Here's how the part is built. I have some questions about the finished solid (model axes, mm). A direction names the side the tool comes from. Round coordinates to 2 decimals unless told otherwise and drop trailing zeros. Write each loop counter-clockwise with the first axis right and the second up, starting at its lowest first coordinate (ties: lowest second). Pieces come first, ordered by that corner, then holes. Notation, with made-up numbers: M 53.25,-37.5 L 59.25,-37.5 A30 cw 59.25,-12.5 Z; hole C 20.5,-3.75 d8. An arc over 180 degrees is marked long. Use one line per item in the form item = value. Start each with the question number.
Q1. I want a section at A-A on z = -9.5. State how many separate pieces and enclosed holes the cut face has, and give its area (3 significant figures).
Q2. We'd pull the mould along Y, two halves only. Please class faces 3 (the face through (-16, 20, -6.35)), 4 (the face through (49.88, 16.57, -4.47)), 5 (the face through (-107.95, -1, 0)), 6 (the face through (-2, 38.1, 0)): +Y half, -Y half, draft (parallel to the pull), parting line (faces both ways), or undercut.
Q3. I want a section at C-C on x = 21. List the corners of the cut face in (y, z) for me (3 decimals), and give its area (3 significant figures).
Q4. I'm going to push flat-ended pins straight in: pin 1 Ø8.5 at (x, y) = (-56.11, -22.45) entering from +Z; pin 2 Ø15.5 at (x, y) = (47, 12.5) entering from -Z. Where does each tip first touch, or does it pass through?
Q5. I want a section at B-B on x = 95.25. List the corners of the cut face in (y, z) for me, and give its area (3 significant figures).
Q6. I want a section at D-D on y = -25.4. List the corners of the cut face in (x, z) for me, and give its area (3 significant figures).
Q7. For faces 1 (the face through (4.58, -29.31, -9.48)), 2 (the face through (89.384, 22.968, -0.178)), which set-ups out of +Z, -Z, +X, -X, +Y, -Y let a thin tool reach every point of the face, with its end or its side?
Q8. I need wall thicknesses on line 1 along X through (y, z) = (-8, -5.25); line 2 along X through (y, z) = (8, -2.5); line 3 along X through (y, z) = (-25.5, -2.5). Which ranges of each line are inside material? Lowest first, please. Write a range as from..to.
```python
from build123d import *

# Parameters (mm, degrees)
SKETCH1_W           = 215.9
SKETCH1_H           = 76.2
BOSS_EXTRUDE1_DEPTH = 12.7
SKETCH2_R           = 5.159375
SKETCH2_R_2         = 6.985
BOSS_EXTRUDE2_DEPTH = 9.525
SKETCH3_R           = 5.159375
BOSS_EXTRUDE3_DEPTH = 9.525
CUT_EXTRUDE1_DEPTH  = 3.81
LPATTERN1_COUNT     = 2
LPATTERN1_PITCH     = 67.31
SKETCH5_R           = 13.335
CUT_EXTRUDE2_DEPTH  = 2.54
SKETCH6_R           = 6.35
CUT_EXTRUDE3_DEPTH  = 118.260276735
SKETCH7_R           = 20.6502
CUT_EXTRUDE4_DEPTH  = 116.571744492


with BuildPart() as part:
    # Sketch1 → Boss-Extrude1 (new, symmetric)
    with BuildSketch(Plane.XY):
        Rectangle(SKETCH1_W, SKETCH1_H)
        with BuildLine():
            ThreePointArc((-52.148499203, -31.128702045), (-62.84981265, -29.19481265), (-64.783702045, -18.493499203))
            Line((-64.783702045, -18.493499203), (-52.443985877, 8.56765836))
            ThreePointArc((-52.443985877, 8.56765836), (-48.256896453, 14.601896453), (-42.22265836, 18.788985877))
            Line((-42.22265836, 18.788985877), (-15.161500797, 31.128702045))
            ThreePointArc((-15.161500797, 31.128702045), (-6.045595474, 30.472789203), (-1.666659697, 22.450640303))
            ThreePointArc((-1.666659697, 22.450640303), (-1.884046645, 20.42592158), (-2.526297955, 18.493499203))
            Line((-2.526297955, 18.493499203), (-14.866014123, -8.56765836))
            ThreePointArc((-14.866014123, -8.56765836), (-19.053103547, -14.601896453), (-25.08734164, -18.788985877))
            Line((-25.08734164, -18.788985877), (-52.148499203, -31.128702045))
        make_face(mode=Mode.SUBTRACT)
        with BuildLine():
            Line((64.783702045, 18.493499203), (52.443985877, -8.56765836))
            ThreePointArc((52.443985877, -8.56765836), (48.256896453, -14.601896453), (42.22265836, -18.788985877))
            Line((42.22265836, -18.788985877), (15.161500797, -31.128702045))
            ThreePointArc((15.161500797, -31.128702045), (4.46018735, -29.19481265), (2.526297955, -18.493499203))
            Line((2.526297955, -18.493499203), (14.866014123, 8.56765836))
            ThreePointArc((14.866014123, 8.56765836), (19.053103547, 14.601896453), (25.08734164, 18.788985877))
            Line((25.08734164, 18.788985877), (52.148499203, 31.128702045))
            ThreePointArc((52.148499203, 31.128702045), (61.264404526, 30.472789203), (65.643340303, 22.450640303))
            ThreePointArc((65.643340303, 22.450640303), (65.425953355, 20.42592158), (64.783702045, 18.493499203))
        make_face(mode=Mode.SUBTRACT)
    extrude(amount=BOSS_EXTRUDE1_DEPTH, both=True)

    # Sketch2 → Boss-Extrude2 (add)
    with BuildSketch(Plane.XY.offset(12.7)):
        with BuildLine():
            Line((-64.783702045, -18.493499203), (-52.443985877, 8.56765836))
            ThreePointArc((-52.443985877, 8.56765836), (-48.256896453, 14.601896453), (-42.22265836, 18.788985877))
            Line((-42.22265836, 18.788985877), (-15.161500797, 31.128702045))
            ThreePointArc((-15.161500797, 31.128702045), (-4.46018735, 29.19481265), (-2.526297955, 18.493499203))
            Line((-2.526297955, 18.493499203), (-14.866014123, -8.56765836))
            ThreePointArc((-14.866014123, -8.56765836), (-19.053103547, -14.601896453), (-25.08734164, -18.788985877))
            Line((-25.08734164, -18.788985877), (-52.148499203, -31.128702045))
            ThreePointArc((-52.148499203, -31.128702045), (-62.84981265, -29.19481265), (-64.783702045, -18.493499203))
        make_face()
        with Locations((-11.204359697, 22.450640303)):
            Circle(SKETCH2_R, mode=Mode.SUBTRACT)
        with Locations((-56.105640303, -22.450640303)):
            Circle(SKETCH2_R, mode=Mode.SUBTRACT)
        with Locations((-33.655, 0)):
            Circle(SKETCH2_R_2, mode=Mode.SUBTRACT)
    boss_extrude2 = extrude(amount=-BOSS_EXTRUDE2_DEPTH)

    # Sketch3 → Boss-Extrude3 (add)
    with BuildSketch(Plane(origin=(0, 0, 3.175), x_dir=(-1, 0, 0), z_dir=(0, 0, -1))):
        with BuildLine():
            ThreePointArc((14.866014123, -8.56765836), (19.053103547, 14.601896453), (42.22265836, 18.788985877))
            Line((42.22265836, 18.788985877), (15.161500797, 31.128702045))
            ThreePointArc((15.161500797, 31.128702045), (4.46018735, 29.19481265), (2.526297955, 18.493499203))
            Line((2.526297955, 18.493499203), (14.866014123, -8.56765836))
        make_face()
        with Locations(Location((11.204359697, 22.450640303, 0), (0, 0, 180))):
            Circle(SKETCH3_R, mode=Mode.SUBTRACT)
        with BuildLine():
            Line((64.783702045, -18.493499203), (52.443985877, 8.56765836))
            ThreePointArc((52.443985877, 8.56765836), (53.834532653, 4.383745196), (54.3052, 0))
            ThreePointArc((54.3052, 0), (44.824308425, -17.368860335), (25.08734164, -18.788985877))
            Line((25.08734164, -18.788985877), (52.148499203, -31.128702045))
            ThreePointArc((52.148499203, -31.128702045), (62.84981265, -29.19481265), (64.783702045, -18.493499203))
        make_face()
        with Locations(Location((56.105640303, -22.450640303, 0), (0, 0, 180))):
            Circle(SKETCH3_R, mode=Mode.SUBTRACT)
    boss_extrude3 = extrude(amount=BOSS_EXTRUDE3_DEPTH)

    # Sketch4 → Cut-Extrude1 (cut)
    with BuildSketch(Plane(origin=(0, 0, -6.35), x_dir=(-1, 0, 0), z_dir=(0, 0, -1))):
        with BuildLine():
            ThreePointArc((32.621288713, 23.167149523), (17.257052323, 16.397947677), (10.487850477, 1.033711287))
            Line((10.487850477, 1.033711287), (14.866014123, -8.56765836))
            ThreePointArc((14.866014123, -8.56765836), (19.053103547, 14.601896453), (42.22265836, 18.788985877))
            Line((42.22265836, 18.788985877), (32.621288713, 23.167149523))
        make_face()
        with BuildLine():
            Line((25.08734164, -18.788985877), (34.688711287, -23.167149523))
            ThreePointArc((34.688711287, -23.167149523), (50.052947677, -16.397947677), (56.822149523, -1.033711287))
            Line((56.822149523, -1.033711287), (52.443985877, 8.56765836))
            ThreePointArc((52.443985877, 8.56765836), (53.834532653, 4.383745196), (54.3052, 0))
            ThreePointArc((54.3052, 0), (44.824308425, -17.368860335), (25.08734164, -18.788985877))
        make_face()
    cut_extrude1 = extrude(amount=-CUT_EXTRUDE1_DEPTH, mode=Mode.SUBTRACT)

    # LPattern1: Boss-Extrude2, Boss-Extrude3, Cut-Extrude1 ×2
    with Locations(*[(i * LPATTERN1_PITCH, 0, 0) for i in range(1, LPATTERN1_COUNT)]):
        add(boss_extrude2)
        add(boss_extrude3)
        add(cut_extrude1, mode=Mode.SUBTRACT)

    # Sketch5 → Cut-Extrude2 (cut)
    with BuildSketch(Plane(origin=(0, 0, 3.175), x_dir=(-1, 0, 0), z_dir=(0, 0, -1))):
        with Locations((33.655, 0)):
            Circle(SKETCH5_R)
        with Locations((-33.655, 0)):
            Circle(SKETCH5_R)
    extrude(amount=-CUT_EXTRUDE2_DEPTH, mode=Mode.SUBTRACT)

    # Sketch6 → Cut-Extrude3 (cut, through all)
    with BuildSketch(Plane(origin=(0, 0, -12.7), x_dir=(-1, 0, 0), z_dir=(0, 0, -1))):
        with Locations((-95.25, 25.4)):
            Circle(SKETCH6_R)
        with Locations((-95.25, -25.4)):
            Circle(SKETCH6_R)
        with Locations(Location((95.25, -25.4, 0), (0, 0, 180))):
            Circle(SKETCH6_R)
        with Locations(Location((95.25, 25.4, 0), (0, 0, 180))):
            Circle(SKETCH6_R)
    extrude(amount=-CUT_EXTRUDE3_DEPTH, mode=Mode.SUBTRACT)

    # Sketch7 → Cut-Extrude4 (cut, through all)
    with BuildSketch(Plane(origin=(0, 0, 3.175), x_dir=(-1, 0, 0), z_dir=(0, 0, -1))):
        with Locations((-33.655, 0)):
            Circle(SKETCH7_R)
        with Locations((33.655, 0)):
            Circle(SKETCH7_R)
    extrude(amount=-CUT_EXTRUDE4_DEPTH, mode=Mode.SUBTRACT)


solid = part.part
```
Reported:
q1.separate_pieces = 1
q1.enclosed_holes = 6
q1.area = 11,300 mm^2
q2.face_3 = undercut
q2.face_4 = undercut
q2.face_5 = draft
q2.face_6 = +Y half
q3.outline = M -38.1,-12.7 L -28.466,-12.7 L -28.466,-6.35 L -19.433,-6.35 L -19.433,-2.54 L -16.318,-2.54 L -16.318,12.7 L -38.1,12.7 Z; M 16.318,-12.7 L 38.1,-12.7 L 38.1,12.7 L 16.318,12.7 Z
q3.area = 1,020 mm^2
q4.pin_1 = through
q4.pin_2 = -6.35
q5.outline = M -38.1,-12.7 L -31.75,-12.7 L -31.75,12.7 L -38.1,12.7 Z; M -19.05,-12.7 L 19.05,-12.7 L 19.05,12.7 L -19.05,12.7 Z; M 31.75,-12.7 L 38.1,-12.7 L 38.1,12.7 L 31.75,12.7 Z
q5.area = 1,290 mm^2
q6.outline = M -107.95,-12.7 L -101.6,-12.7 L -101.6,12.7 L -107.95,12.7 Z; M -88.9,-12.7 L -65.18,-12.7 L -65.18,-6.35 L -60.34,-6.35 L -60.34,12.7 L -88.9,12.7 Z; M -51.87,-6.35 L -39.59,-6.35 L -39.59,-12.7 L 2.13,-12.7 L 2.13,-6.35 L 6.97,-6.35 L 6.97,12.7 L -51.87,12.7 Z; M 15.44,-6.35 L 27.72,-6.35 L 27.72,-12.7 L 88.9,-12.7 L 88.9,12.7 L 15.44,12.7 Z; M 101.6,-12.7 L 107.95,-12.7 L 107.95,12.7 L 101.6,12.7 Z
q6.area = 4,190 mm^2
q7.face_1 = -Z
q7.face_2 = +Z, -Z
q8.line_1 = -107.95..-55.42, -14.61..11.89, 52.7..107.95
q8.line_2 = -107.95..-52.69, -14.62..14.62, 52.69..107.95
q8.line_3 = -107.95..-101.6, -88.9..-60.27, -51.94..7.04, 15.37..88.9, 101.6..107.95
